Input: part model. Units: mm. Frame: model coordinates. A direction names the side the tool comes from. Give positions to 0.01 mm unless a question says otherwise; leave off trailing zeros. Order: outer loops, then holes, each group sorted by start corner. A loop starts at its lowest first (then second) coordinate and runs counter-clockwise, first axis right, second up. Notation, with made-up numbers: M 8.5,-3.5 L 40.5,-3.5 A21 cw 40.5,34.5 Z; hole C 89.5,54 d9. An arc over 180 degrees is marked long. Use a Markdown table: item, result.
Autodesk Inventor part; units mm, degrees
ref_plane "YZ Plane" through (0, 0, 0) normal (1, 0, 0) x (0, 1, 0)
ref_plane "XZ Plane" through (0, 0, 0) normal (0, 1, 0) x (-1, 0, 0)
ref_plane "XY Plane" through (0, 0, 0) normal (0, 0, 1) x (1, 0, 0)
sketch "スケッチ1" plane through (0, 0, 0) normal (0, 1, 0) x (-1, 0, 0)
  circle A0 centre (0, 0) radius 2.75
  dimension "d0" = 5.5
extrude "押し出し1" add sketch "スケッチ1" along normal blind 3
sketch "スケッチ2" plane through (0, 0, 0) normal (0, -1, 0) x (1, 0, 0)
  circle A0 centre (0, 0) radius 1.5
  dimension "d3" = 3
extrude "押し出し2" add sketch "スケッチ2" along normal blind 5
fillet "フィレット1" radius 0.5 1 edges at (2.75, 3, 0)
fillet "フィレット1" radius 0.2 1 edges at (2.75, 0, 0)
sketch "スケッチ3" plane through (0, 3, 0) normal (0, 1, 0) x (1, 0, 0)
  line L0 (0, 1.4434) -> (-1.25, 0.7217)
  line L1 (-1.25, 0.7217) -> (-1.25, -0.7217)
  line L2 (-1.25, -0.7217) -> (0, -1.4434)
  line L3 (0, -1.4434) -> (1.25, -0.7217)
  line L4 (1.25, -0.7217) -> (1.25, 0.7217)
  line L5 (1.25, 0.7217) -> (0, 1.4434)
  line L6 (0, 1.4434) -> (0, -1.4434) construction
  circle A0 centre (0, 0) radius 1.4434 construction
  dimension "d12" = 2.5
extrude "押し出し3" cut sketch "スケッチ3" against normal blind 2
thread "ねじ1"
properties part number "M3-CapScrew"
1) Mould query, pull axis Z, two halves, no side actions, for faces 3 (the face through (-2, 0, 0)), 4 (the face through (1.25, 2, 0)), 5 (the face through (-1.5, -2.46, -0.07)), 6 (the face through (0, 1, 0)). Classes: released by +Z, released by -Z, zero draft, split by the parting line, or undercut.
Response values:
| item | result |
|---|---|
| face 3 | zero draft |
| face 4 | undercut |
| face 5 | split by the parting line |
| face 6 | undercut |
2) First-contact query: pin 1 Ø2 at (x, y) = (-1, -0.5) entering from -Z. Flat tip, straight axial feed; report the tip coordinate or a pass-through.
Response values:
| item | result |
|---|---|
| pin 1 | stops at z = -2.74 |
3) Material intervals for line 1 (Y direction, x = -1, z = 0.4); line 2 (X direction, y = 2, z = -0.75); line 3 (X direction, y = 1.75, z = 0.3), sorted ascending. Write a range as from..to.
Response values:
| item | result |
|---|---|
| line 1 | y = -5..1 |
| line 2 | x = -2.65..-1.2, 1.2..2.65 |
| line 3 | x = -2.73..-1.25, 1.25..2.73 |
4) Reachability of faces 1 (the face through (0, -5, 0)), 2 (the face through (-1.25, 2, 0)) from +Z, -Z, +X, -X, +Y, -Y: full face, straight path, thin tool, end or side. Return the list, or none.
Response values:
| item | result |
|---|---|
| face 1 | +Z, -Z, +X, -X, -Y |
| face 2 | +Y |
5) Cut plane B-B on z = 0. Return loops of the section in (x, y).
Response values:
| item | result |
|---|---|
| outline | M -2.75,0.2 A0.2 ccw -2.55,0 L -1.5,0 L -1.5,-5 L 1.5,-5 L 1.5,0 L 2.55,0 A0.2 ccw 2.75,0.2 L 2.75,2.5 A0.5 ccw 2.25,3 L 1.25,3 L 1.25,1 L -1.25,1 L -1.25,3 L -2.25,3 A0.5 ccw -2.75,2.5 Z |
6) Cut plane A-A on y = 2. Return loops of the section in (x, z).
Response values:
| item | result |
|---|---|
| outline | C 0,0 d5.5; hole M -1.25,-0.72 L 0,-1.44 L 1.25,-0.72 L 1.25,0.72 L 0,1.44 L -1.25,0.72 Z |
7) Cut plane C-C on y = -2.75. Return loops of the section in (x, z).
Response values:
| item | result |
|---|---|
| outline | C 0,0 d3 |
